Work out the finished part from the listing and answer in its coordinate system (mm). A direction names the side the tool comes from. Coordinates: 2 decimals unless noted, no trailing zeros. Use a Markdown table: item, result. Add a question column.
(1) Given pin 1 Ø1.2 at (x, z) = (-1.5, 2.5) entering from +Y; pin 2 Ø1 at (y, z) = (38.5, 1.5) entering from -X; pin 3 Ø1.1 at (x, z) = (-3.5, 1.5) entering from -Y; pin 4 Ø1.8 at (x, y) = (14, 5) entering from -Z, each flat-ended and moving along its own axis, determine where each tip first touches the part or whether it passes through.
(2) A tool of negligible diameter and unlimited length cuts with its end or side. For faces 4 (the face through (4, 0, 6)), 5 (the face through (10, 104, 3)), 6 (the face through (5, 74, 0)), 7 (the face through (16.797, 1.141, 2.535)), 8 (the face through (0, 104, 3)), from which of +Z, -Z, +X, -X, +Y, -Y can it reach the whole face along a straight path? Write none if from no direction.
(3) Find the intervals of material crossed by line 1 (Y direction, x = -4, z = 1.5); line 2 (X direction, y = 89, z = 3.5); line 3 (Y direction, x = 0.5, z = 5.25), in increasing order. Write a range as from..to.
(4) For a pull along Z with two mould halves and no side action, classify faces 1 (the face through (5, -1, 5)), 2 (the face through (16.859, 8.797, 2.535)), 3 (the face through (4.77, 2.23, 6.91)) as released by +Z, released by -Z, zero draft, split by the parting line, or undercut.
from build123d import *

# Parameters (mm, degrees)
SKETCH1_W           = 10
SKETCH1_H           = 10
BOSS_EXTRUDE1_DEPTH = 200
FILLET1_SIZE        = 5
SKETCH2_R           = 1.5
CUT_EXTRUDE1_DEPTH  = 201.499376667
FILLET2_R           = 1
SKETCH4_W           = 8
SKETCH4_H           = 10
BOSS_EXTRUDE2_DEPTH = 5
SKETCH5_W           = 10
SKETCH5_H           = 5
BOSS_EXTRUDE3_DEPTH = 8
FILLET3_R           = 4
FILLET4_R           = 3
SKETCH6_R           = 1.5
CUT_EXTRUDE3_DEPTH  = 201.870605219
SKETCH7_R           = 0.75
CUT_EXTRUDE4_DEPTH  = 8


with BuildPart() as part:
    # Sketch1 → Boss-Extrude1 (new body)
    with BuildSketch(Plane(origin=(0, 0, 0), x_dir=(1, 0, 0), z_dir=(0, 1, 0))):
        with Locations((5, -5)):
            Rectangle(SKETCH1_W, SKETCH1_H)
    extrude(amount=BOSS_EXTRUDE1_DEPTH)

    # Fillet1
    # a fillet whose section is not a circle: 5 mm, written as the material it takes off along each edge
    with BuildSketch(Plane(origin=(0, -12.5, 10), x_dir=(1, 0, 0), z_dir=(0, 1, 0)), Plane(origin=(10, -12.5, 10), x_dir=(0, 0, -1), z_dir=(0, 1, 0))) as fillet1_piece_1:
        with BuildLine():
            Bezier((FILLET1_SIZE, 0), (0, 0), (0, FILLET1_SIZE), weights=[1, 0.052631579, 1])
            Line((0, FILLET1_SIZE), (0, 0))
            Line((0, 0), (FILLET1_SIZE, 0))
        make_face()
    extrude(amount=225, mode=Mode.SUBTRACT)

    # Sketch2 → Cut-Extrude1 (cut, through all)
    with BuildSketch(Plane(origin=(0, 0, 0), x_dir=(-1, 0, 0), z_dir=(0, -1, 0))):
        with Locations((-5, -10)):
            Circle(SKETCH2_R)
    extrude(amount=-CUT_EXTRUDE1_DEPTH, mode=Mode.SUBTRACT)

    # Fillet2
    fillet2_edges = [part.edges().sort_by_distance(p)[0] for p in [
        (3.843309936, 100, 9.044977437),
        (6.156690064, 100, 9.044977437),
    ]]
    fillet(fillet2_edges, radius=FILLET2_R)

    # Sketch4 → Boss-Extrude2 (add)
    with BuildSketch(Plane(origin=(0, 0, 0), x_dir=(-1, 0, 0), z_dir=(0, 0, -1))):
        with Locations((4, 5)):
            Rectangle(SKETCH4_W, SKETCH4_H)
        with Locations((-14, 5)):
            Rectangle(SKETCH4_W, SKETCH4_H)
    extrude(amount=-BOSS_EXTRUDE2_DEPTH)

    # Sketch5 → Boss-Extrude3 (add)
    with BuildSketch(Plane(origin=(0, 0, 0), x_dir=(-1, 0, 0), z_dir=(0, -1, 0))):
        with Locations((-5, -2.5)):
            Rectangle(SKETCH5_W, SKETCH5_H)
    extrude(amount=BOSS_EXTRUDE3_DEPTH)

    # Fillet3
    fillet3_edges = [part.edges().sort_by_distance(p)[0] for p in [
        (18, 10, 2.5),
        (18, 0, 2.5),
        (10, -8, 2.5),
        (0, -8, 2.5),
        (-8, 10, 2.5),
        (-8, 0, 2.5),
    ]]
    fillet(fillet3_edges, radius=FILLET3_R)

    # Fillet4
    # the kernel refuses this fillet: 3 mm, written as the material it adds along each edge
    with BuildSketch(Plane(origin=(10, 0, 0), x_dir=(1, 0, 0), z_dir=(0, 0, 1)), Plane(origin=(0, 0, 5), x_dir=(-1, 0, 0), z_dir=(0, 0, -1))) as fillet4_piece_1:
        with BuildLine():
            CenterArc((FILLET4_R, -FILLET4_R), FILLET4_R, 90, 90)
            Line((0, -FILLET4_R), (0, 0))
            Line((0, 0), (FILLET4_R, 0))
        make_face()
    extrude(amount=5)

    # Sketch6 → Cut-Extrude3 (cut, through all)
    with BuildSketch(Plane.XY.offset(5)):
        with Locations((-4, 5)):
            Circle(SKETCH6_R)
        with Locations((14, 5)):
            Circle(SKETCH6_R)
        with Locations((5, -4)):
            Circle(SKETCH6_R)
    extrude(amount=-CUT_EXTRUDE3_DEPTH, mode=Mode.SUBTRACT)

    # Sketch7 → Cut-Extrude4 (cut)
    with BuildSketch(Plane(origin=(0, 2.349231552, 1.644949642), x_dir=(-1, 0, 0), z_dir=(0, 0.8191520442889949, 0.5735764363510416))):
        with Locations(Location((-5, 5.095760221, 0), (0, 0, 270))):
            Circle(SKETCH7_R)
    extrude(amount=CUT_EXTRUDE4_DEPTH, mode=Mode.SUBTRACT)


solid = part.part
Model answer:
| question | item | result |
|---|---|---|
| 1 | pin 1 | y = 10 |
| 1 | pin 2 | x = 0 |
| 1 | pin 3 | y = 0 |
| 1 | pin 4 | through |
| 2 | face 4 | +Z, +X, -X, -Y |
| 2 | face 5 | +Z, -Z, +X, +Y |
| 2 | face 6 | -Z, +X, -X, +Y, -Y |
| 2 | face 7 | +Z, -Z, +X, -Y |
| 2 | face 8 | +Z, -Z, -X, +Y |
| 3 | line 1 | 0..3.5, 6.5..10 |
| 3 | line 2 | 0..10 |
| 3 | line 3 | 0..200 |
| 4 | face 1 | released by +Z |
| 4 | face 2 | zero draft |
| 4 | face 3 | undercut |
